Read the model definition and answer for the solid it produces. Units are mm, in the model's axes. Give positions to 0.01 mm unless a question says otherwise; leave off trailing zeros. Write each loop counter-clockwise with the first axis right and the second up, starting at its lowest first coordinate (ties: lowest second). Pieces come first, ordered by that corner, then holes. Notation, with made-up numbers: (-5, 67) -> (44, 67) arc R29 ccw to (44, 87) -> close; hole circle Ø11 at (12, 11). An arc over 180 degrees is marked (long way). Use a Markdown table: item, result.
from build123d import *

# Parameters (mm, degrees)
SKETCH1_R           = 2
BOSS_EXTRUDE1_DEPTH = 3
SKETCH3_R           = 2
CUT_EXTRUDE1_DEPTH  = 3


with BuildPart() as part:
    # Sketch1 → Boss-Extrude1 (new body)
    with BuildSketch(Plane.XY):
        with BuildLine():
            Line((0, 18), (-70, 18))
            ThreePointArc((-70, 18), (-88, 0), (-70, -18))
            Line((-70, -18), (0, -18))
            ThreePointArc((0, -18), (18, 0), (0, 18))
        make_face()
        Circle(SKETCH1_R, mode=Mode.SUBTRACT)
    extrude(amount=BOSS_EXTRUDE1_DEPTH)

    # Sketch3 → Cut-Extrude1 (cut)
    with BuildSketch(Plane.XY.offset(3)):
        with Locations((10, 0)):
            Circle(SKETCH3_R)
    extrude(amount=-CUT_EXTRUDE1_DEPTH, mode=Mode.SUBTRACT)


solid = part.part
Item 1: A cutting plane is placed at A-A (y = 0). Give the vertices of the cut face in (x, z).
Return value:
| item | result |
|---|---|
| outline | (-88, 0) -> (-2, 0) -> (-2, 3) -> (-88, 3) -> close; (2, 0) -> (8, 0) -> (8, 3) -> (2, 3) -> close; (12, 0) -> (18, 0) -> (18, 3) -> (12, 3) -> close |
Item 2: Straight lines are drawn through the part: line 1 along Y through (x, z) = (10, 0.6); line 2 along X through (y, z) = (4, 0.95); line 3 along Y through (x, z) = (-74, 0.55). For each, find the intervals that lie inside material, in ascending order. Write a range as [from, to].
Return value:
| item | result |
|---|---|
| line 1 | [-14.97, -2], [2, 14.97] |
| line 2 | [-87.55, 17.55] |
| line 3 | [-17.55, 17.55] |
Item 3: This flat-tipped pin is pushed along its axis until it touches: P1, Ø1, axis at y = -0.5, z = 1.5, coming from the +X side. Where does it stop, or does it pass through?
Return value:
| item | result |
|---|---|
| P1 | x = 18 |
Item 4: A cutting plane is placed at C-C (z = 2.45). Give the vertices of the cut face in (x, y), then the cut area to 3 significant figures.
Return value:
| item | result |
|---|---|
| outline | (-70, -18) -> (0, -18) arc R18 ccw to (0, 18) -> (-70, 18) arc R18 ccw to start; hole circle Ø4 at (0, 0); hole circle Ø4 at (10, 0) |
| area | 3,510 mm^2 |
Item 5: A cutting plane is placed at B-B (x = 10). Give the vertices of the cut face in (y, z).
Return value:
| item | result |
|---|---|
| outline | (-14.97, 0) -> (-2, 0) -> (-2, 3) -> (-14.97, 3) -> close; (2, 0) -> (14.97, 0) -> (14.97, 3) -> (2, 3) -> close |
Item 6: A cutting plane is placed at D-D (y = -7). Give the vertices of the cut face in (x, z), then the cut area to 3 significant figures.
Return value:
| item | result |
|---|---|
| outline | (-86.58, 0) -> (16.58, 0) -> (16.58, 3) -> (-86.58, 3) -> close |
| area | 309 mm^2 |
Item 7: For a pull along X with two mould halves and no side action, classify faces 1 (the face through (-88, 0, 1)), 2 (the face through (18, 0, 1)), 3 (the face through (8.4, -1.2, 1.5)), 4 (the face through (-35, 18, 1)) as +X half, -X half, draft (parallel to the pull), parting line (faces both ways), or undercut.
Return value:
| item | result |
|---|---|
| face 1 | -X half |
| face 2 | +X half |
| face 3 | undercut |
| face 4 | draft |
